Could you check a few things on this model? Use its own coordinates, in mm. A direction names the side the tool comes from. Round coordinates to 2 decimals unless told otherwise and drop trailing zeros. Loops run counter-clockwise (first coordinate to the right, second up) from the corner with the lowest first, then second, coordinate; pieces in that order, holes last.
from build123d import *

# Parameters (mm, degrees)
SKETCH2_W           = 40
SKETCH2_H           = 3
BOSS_EXTRUDE1_DEPTH = 4
SKETCH3_W           = 40
SKETCH3_H           = 3
BOSS_EXTRUDE2_DEPTH = 16
SKETCH4_R           = 3
BOSS_EXTRUDE3_DEPTH = 16
SKETCH5_R           = 1.5
CUT_EXTRUDE1_DEPTH  = 37
SKETCH6_R           = 1.5
CUT_EXTRUDE2_DEPTH  = 4
FILLET1_R           = 4
FILLET2_R           = 2


with BuildPart() as part:
    # Sketch2 → Boss-Extrude1 (new body)
    with BuildSketch(Plane(origin=(0, 0, 0), x_dir=(0, 0, -1), z_dir=(1, 0, 0))):
        Polygon((-5, 15), (-10, 1.5), (10, 1.5), (5, 15), align=None)
        Rectangle(SKETCH2_W, SKETCH2_H)
    extrude(amount=BOSS_EXTRUDE1_DEPTH)

    # Sketch3 → Boss-Extrude2 (add)
    with BuildSketch(Plane(origin=(4, 0, 0), x_dir=(0, 0, -1), z_dir=(1, 0, 0))):
        Rectangle(SKETCH3_W, SKETCH3_H)
    extrude(amount=BOSS_EXTRUDE2_DEPTH)

    # Sketch4 → Boss-Extrude3 (add)
    with BuildSketch(Plane.ZY):
        with Locations((0, 9)):
            Circle(SKETCH4_R)
    extrude(amount=BOSS_EXTRUDE3_DEPTH)

    # Sketch5 → Cut-Extrude1 (cut, through all)
    with BuildSketch(Plane.ZY.offset(16)):
        with Locations((0, 9)):
            Circle(SKETCH5_R)
    extrude(amount=-CUT_EXTRUDE1_DEPTH, mode=Mode.SUBTRACT)

    # Sketch6 → Cut-Extrude2 (cut, through all)
    with BuildSketch(Plane(origin=(0, 1.5, 0), x_dir=(1, 0, 0), z_dir=(0, 1, 0))):
        with BuildLine():
            ThreePointArc((18.5, 15), (17, 16.5), (15.5, 15))
            Line((15.5, 15), (17, 15))
            Line((17, 15), (17, 13.5))
            ThreePointArc((17, 13.5), (18.060660172, 13.939339828), (18.5, 15))
        make_face()
        with BuildLine():
            Line((17, 15), (15.5, 15))
            ThreePointArc((15.5, 15), (15.939339828, 13.939339828), (17, 13.5))
            Line((17, 13.5), (17, 15))
        make_face()
        with BuildLine():
            ThreePointArc((18.5, -15), (18.060660172, -13.939339828), (17, -13.5))
            Line((17, -13.5), (17, -15))
            Line((17, -15), (15.5, -15))
            ThreePointArc((15.5, -15), (17, -16.5), (18.5, -15))
        make_face()
        with BuildLine():
            Line((17, -15), (17, -13.5))
            ThreePointArc((17, -13.5), (15.939339828, -13.939339828), (15.5, -15))
            Line((15.5, -15), (17, -15))
        make_face()
        with BuildLine():
            ThreePointArc((4.5, -15), (4.060660172, -13.939339828), (3, -13.5))
            Line((3, -13.5), (3, -15))
            Line((3, -15), (4.5, -15))
        make_face()
        with BuildLine():
            Line((3, -15), (3, -13.5))
            ThreePointArc((3, -13.5), (1.939339828, -16.060660172), (4.5, -15))
            Line((4.5, -15), (3, -15))
        make_face()
        with Locations((3, 15)):
            Circle(SKETCH6_R)
    extrude(amount=-CUT_EXTRUDE2_DEPTH, mode=Mode.SUBTRACT)

    # Fillet1
    fillet1_edges = [part.edges().sort_by_distance(p)[0] for p in [
        (4, 1.5, 0),
    ]]
    fillet(fillet1_edges, radius=FILLET1_R)

    # Fillet2
    fillet2_edges = [part.edges().sort_by_distance(p)[0] for p in [
        (0, 9, -3),
    ]]
    fillet(fillet2_edges, radius=FILLET2_R)


solid = part.part
Item 1: If we section it at D-D, the plane x = 8.5: Please give me the cut outline in (y, z), then the cut area to 3 significant figures.
Results list:
outline: (-1.5, -20) - (1.5, -20) - (1.5, 20) - (-1.5, 20) - close
area: 120 mm2
Item 2: Will these pins go through, and if not, where does the flat tip stop? pin 1 (6 mm diameter, centred on x = 13.5, z = -15.5, fed in from +Y); pin 2 (1 mm diameter, centred on x = -4, y = 11.5, fed in from -Z); pin 3 (5 mm diameter, centred on y = 8.5, z = -2, fed in from +X); pin 4 (2.5 mm diameter, centred on y = 9, z = 0, fed in from -X).
Results list:
pin 1: stops at y = 1.5
pin 2: stops at z = -2.24
pin 3: stops at x = 4
pin 4: passes through
Item 3: For faces 4 (the flat face through (10, -1.5, 0)), 5 (the flat face through (4, 11, 0)), which set-ups out of +Z, -Z, +X, -X, +Y, -Y let a thin tool reach every point of the face, with its end or its side?
Results list:
face 4: +Z, -Z, +X, -X, -Y
face 5: +Z, -Z, +X, +Y
Item 4: We'd pull the mould along Z, two halves only. Please class faces 1 (the flat face through (20, 0, 0)), 2 (the cylindrical face through (4.386, 0.021, -14.425)), 3 (the cylindrical face through (-9, 9, -3)): released by +Z, released by -Z, zero draft, split by the parting line, or undercut.
Results list:
face 1: zero draft
face 2: undercut
face 3: split by the parting line
Item 5: If I drill on line 1 along X through (y, z) = (0.9, 15); line 2 along Z through (x, y) = (3, 0.6); line 3 along Y through (x, z) = (-9, 0), over which ranges is the centre line in solid material (lowest first)?
Results list:
line 1: x = 0 to 1.5, 4.5 to 15.5, 18.5 to 20
line 2: z = -20 to -16.5, -13.5 to 13.5, 16.5 to 20
line 3: y = 6 to 7.5, 10.5 to 12
Item 6: If we section it at B-B, the plane y = 9: Please give me the cut outline in (x, z).
Results list:
outline: (-16, -3) - (-2, -3) arc R2 cw to (0, -5) - (0, -7.22) - (4, -7.22) - (4, -1.5) - (-16, -1.5) - close; (-16, 1.5) - (4, 1.5) - (4, 7.22) - (0, 7.22) - (0, 5) arc R2 cw to (-2, 3) - (-16, 3) - close
Item 7: If we section it at C-C, the plane z = 14.5: Please give me the cut outline in (x, y).
Results list:
outline: (0, -1.5) - (1.59, -1.5) - (1.59, 1.5) - (0, 1.5) - close; (4.41, -1.5) - (15.59, -1.5) - (15.59, 1.5) - (4.41, 1.5) - close; (18.41, -1.5) - (20, -1.5) - (20, 1.5) - (18.41, 1.5) - close
Item 8: If we section it at A-A, the plane z = -14: Please give me the cut outline in (x, y), then the cut area to 3 significant figures.
Results list:
outline: (0, -1.5) - (1.88, -1.5) - (1.88, 1.5) - (0, 1.5) - close; (4.12, -1.5) - (15.88, -1.5) - (15.88, 1.5) - (4.12, 1.5) - close; (18.12, -1.5) - (20, -1.5) - (20, 1.5) - (18.12, 1.5) - close
area: 46.6 mm2
